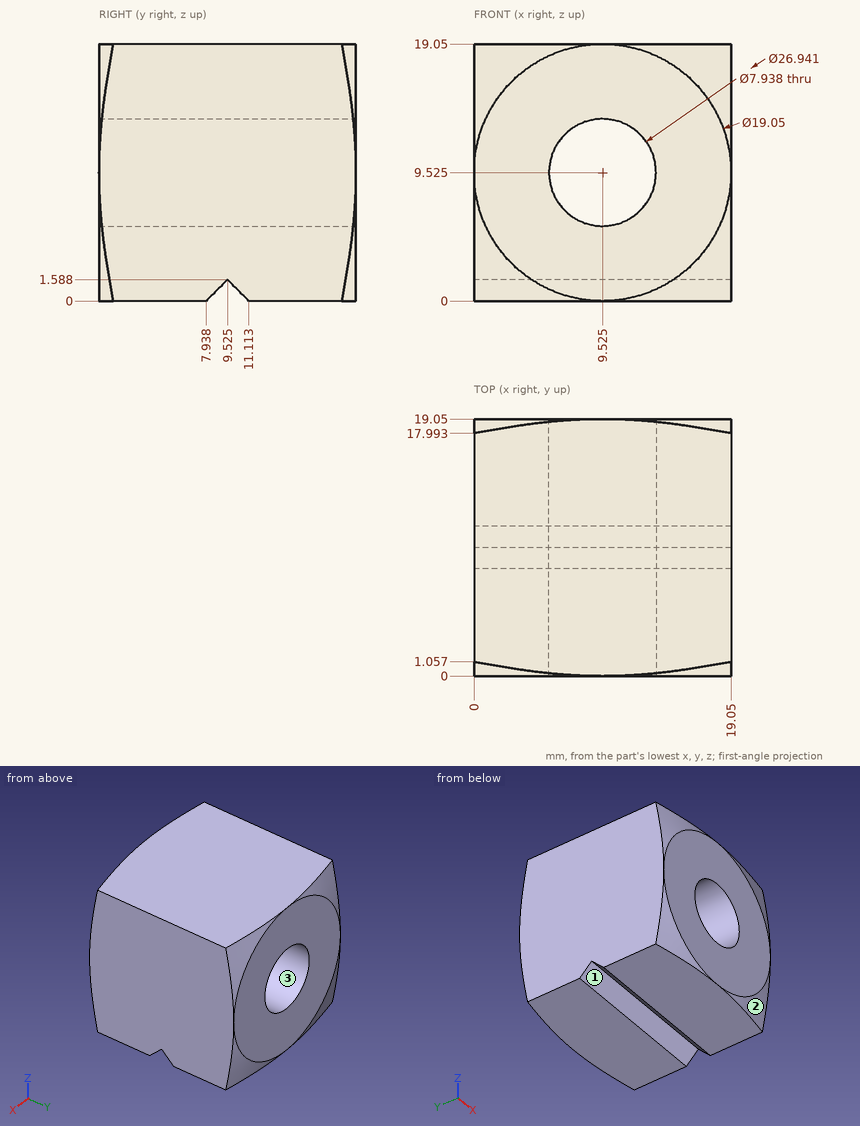
Answer from the drawing. Dimensions are ordinates in mm from the lowest x, y and z of the part. Give positions to 0.01 mm unless a question says otherwise; leave off trailing zeros.
Item 1: Find the intervals of material crossed by line 1 along Z through (x, y) = (11.25, 16); line 2 along Z through (x, y) = (8.75, 3.25); line 3 along X through (y, z) = (14.5, 10.5), in increasing order.
Item 2: This flat-tipped pin is pushed along its axis until it touches: pin 1 Ø2 at (x, z) = (10, 8.5) entering from +Y. Where does it stop, or does it pass through?
Item 3: The mould has two halves that part along X. Classify the marked faces 1, 2 and 3: released by +X, released by -X, zero draft, split by the parting line, or undercut.
Taken from the geometry:
1. line 1: z = 0 to 5.95, 13.1 to 19.05
1. line 2: z = 0 to 5.63, 13.42 to 19.05
1. line 3: x = 0 to 5.68, 13.37 to 19.05
2. pin 1: passes through
3. face 1: zero draft
3. face 2: released by +X
3. face 3: undercut
